Can you work these out from the model? Positions are in its coordinate system, mm. A direction names the side the tool comes from. Give positions to 0.01 mm unless a question says otherwise; leave off trailing zeros. Write each loop counter-clockwise with the first axis right and the second up, starting at its lowest first coordinate (ties: lowest second). Pieces come first, ordered by that corner, then holes. Notation, with made-up numbers: (-16, -9.5) -> (8, -9.5) arc R17 ccw to (8, 11.5) -> close; hole circle Ø5 at (-38.5, 8.25). An arc over 180 degrees is marked (long way). One line per item, written item: value.
Autodesk Inventor part; units mm, degrees
ref_plane "YZ Plane" through (0, 0, 0) normal (1, 0, 0) x (0, 1, 0)
ref_plane "XZ Plane" through (0, 0, 0) normal (0, 1, 0) x (-1, 0, 0)
ref_plane "XY Plane" through (0, 0, 0) normal (0, 0, 1) x (1, 0, 0)
sketch "Sketch1" plane through (0, 0, 0) normal (0, 0, 1) x (1, 0, 0)
  line L0 (-21.1, 10.5) -> (21.1, 10.5)
  line L1 (21.1, 10.5) -> (21.1, -10.5)
  line L2 (21.1, -10.5) -> (-21.1, -10.5)
  line L3 (-21.1, -10.5) -> (-21.1, 10.5)
  line L4 (-21.1, 10.5) -> (21.1, -10.5) construction
  line L5 (21.1, 10.5) -> (-21.1, -10.5) construction
  line L6 (31.1, 20.5) -> (-31.1, 20.5)
  line L7 (-31.1, 20.5) -> (-31.1, -20.5)
  line L8 (-31.1, -20.5) -> (31.1, -20.5)
  line L9 (31.1, -20.5) -> (31.1, 20.5)
  point P0 (0, 0)
  dimension "d0" = 42.2
  dimension "d1" = 21
  dimension "d2" = 10
extrude "Extrusion1" add sketch "Sketch1" along normal blind 9
sketch "Sketch2" plane through (-31.1, -20.5, 0) normal (0, -1, 0) x (1, 0, 0)
  line L0 (62.2, 9) -> (0, 9)
  line L1 (0, 9) -> (75, 9)
  line L2 (75, 9) -> (75, -11)
  line L3 (75, -11) -> (0, -11)
  line L4 (0, -11) -> (0, 9)
  point P0 (31.1, 0)
  dimension "d5" = 75
  dimension "d6" = 20
extrude "Extrusion2" add sketch "Sketch2" along normal blind 5
sketch "Sketch3" plane through (-31.1, 20.5, 0) normal (-1, 0, 0) x (0, 0, 1)
  line L0 (9, -46) -> (-11, -46)
  line L1 (9, -46) -> (-11, -46)
  line L2 (-11, -46) -> (-11, 14)
  line L3 (-11, 14) -> (9, 14)
  line L4 (9, 14) -> (9, -46)
  point P0 (0, -20.5)
  dimension "d9" = 20
  dimension "d10" = 60
extrude "Extrusion3" add sketch "Sketch3" along normal blind 5
sketch "Sketch4" plane through (-31.1, -25.5, 0) normal (0, -1, 0) x (1, 0, 0)
  line L0 (75, 9) -> (75, -11)
  line L1 (75, 2.3333) -> (-5, 2.3333)
  line L2 (-5, -11) -> (-5, 9)
  line L3 (75, -3.6667) -> (-5, -3.6667)
  line L4 (75, 9) -> (-5, 9)
  line L5 (75, 2.3333) -> (75, -3.6667)
  line L6 (-5, 2.3333) -> (-5, -3.6667)
  point P0 (31.1, 0)
  dimension "d13" = 6
  dimension "d14" = 6.6667
extrude "Extrusion4" add sketch "Sketch4" along normal blind 1.5 contours L0 L3 L2 L1
sketch "Sketch5" plane through (-36.1, 20.5, 0) normal (-1, 0, 0) x (0, 0, 1)
  line L0 (2.353, -47.5) -> (2.353, 14)
  line L1 (9, 14) -> (-11, 14)
  line L2 (2.3333, -47.5) -> (-3.6667, -47.5)
  line L3 (-3.6667, -47.5) -> (-3.6667, 14)
  line L4 (-3.6667, 14) -> (2.353, 14)
  line L5 (2.353, -47.5) -> (-3.6667, -47.5)
  point P0 (0, -20.5)
extrude "Extrusion5" add sketch "Sketch5" along normal blind 1.5
sketch "Sketch6" plane through (-37.6, 20.5, 0) normal (-1, 0, 0) x (0, 0, 1)
  line L0 (9, 14) -> (2.353, 14)
  line L1 (0, 0) -> (9, 0)
  line L2 (9, -46) -> (9, 14)
  line L3 (-11, 14) -> (-11, -46)
  point P0 (0, -20.5)
  point P1 (-1, 7)
  dimension "d19" = 14
  dimension "d20" = 20
  dimension "d21" = 10
  dimension "d22" = 7
hole "Hole1" at (-37.6, 27.5, -1) direction (1, 0, 0) diameter 6 end through all counterbore diameter 10 counterbore depth 1.5
sketch "Sketch7" plane through (-31.1, -27, 0) normal (0, -1, 0) x (1, 0, 0)
  line L0 (75, 2.3333) -> (75, 9)
  line L1 (62.2, 0) -> (62.2, 9)
  line L2 (75, -11) -> (-5, -11)
  line L3 (75, 9) -> (-5, 9)
  point P0 (31.1, 0)
  point P1 (68.6, -1)
  dimension "d30" = 12.8
  dimension "d31" = 20
  dimension "d32" = 10
  dimension "d33" = 6.4
hole "Hole2" at (37.5, -27, -1) direction (0, 1, 0) diameter 6 end through all counterbore diameter 10 counterbore depth 1.5
fillet "Fillet1" radius 2 9 edges at (31.1, 20.5, 4.5) (-33.6, 34.5, 9) (-33.6, 34.5, -11) (43.9, -23, 9) (43.9, -23, -11) (0, 10.5, 0) (0, -10.5, 0) (21.1, 0, 0) (-21.1, 0, 0)
properties part number "SuporteRJ45"
1) For faces 5 (the face through (43.33, -23.04, 8.4)), 6 (the face through (0, 14, 0)), 7 (the face through (31.1, -1, 4)), which set-ups out of +Z, -Z, +X, -X, +Y, -Y let a thin tool reach every point of the face, with its end or its side?
Answer list:
face 5: +Z, +X, +Y, -Y
face 6: -Z, +X, +Y
face 7: +Z, -Z, +X, +Y
2) If we section it at C-C (z = -1): Write out the boundary of the cut face in (x, y), and give its area (3 significant figures).
Answer list:
outline: (-37.6, -27) -> (32.5, -27) -> (32.5, -25.5) -> (34.5, -25.5) -> (34.5, -20.5) -> (-31.1, -20.5) -> (-31.1, 24.5) -> (-36.1, 24.5) -> (-36.1, 22.5) -> (-37.6, 22.5) -> close; (-37.6, 32.5) -> (-36.1, 32.5) -> (-36.1, 30.5) -> (-31.1, 30.5) -> (-31.1, 34.5) -> (-37.6, 34.5) -> close; (40.5, -25.5) -> (42.5, -25.5) -> (42.5, -27) -> (43.9, -27) -> (43.9, -20.5) -> (40.5, -20.5) -> close
area: 797 mm^2
3) We'd pull the mould along Y, two halves only. Please class faces 1 (the face through (21.1, 0, 5)), 2 (the face through (-14, -22, -11)), 3 (the face through (-21.67, 0.18, 0.6)), 4 (the face through (43, -27, -1)): released by +Y, released by -Y, zero draft, split by the parting line, or undercut.
Answer list:
face 1: undercut
face 2: zero draft
face 3: undercut
face 4: released by -Y
4) If we section it at B-B (x = 37.5): Write out the boundary of the cut face in (y, z).
Answer list:
outline: (-25.5, -11) -> (-20.5, -11) -> (-20.5, -4) -> (-25.5, -4) -> close; (-25.5, 2) -> (-20.5, 2) -> (-20.5, 9) -> (-25.5, 9) -> close
5) If we section it at A-A (y = 27.5): Write out the boundary of the cut face in (x, z).
Answer list:
outline: (-36.1, -11) -> (-31.1, -11) -> (-31.1, -4) -> (-36.1, -4) -> close; (-36.1, 2) -> (-31.1, 2) -> (-31.1, 9) -> (-36.1, 9) -> close
6) I need wall thicknesses on L1, parallel to Y at x = -6, z = 3.25; L2, parallel to X at y = -23.95, z = -1; L3, parallel to X at y = -9.5, z = 5.75. Which ranges of each line are inside material? Lowest first, please.
Answer list:
L1: y = -25.5 to -10.5, 10.5 to 20.5
L2: x = -37.6 to 34.5, 40.5 to 43.9
L3: x = -36.1 to -21.1, 21.1 to 31.1
7) Will these pins go through, and if not, where does the flat tip stop? pin 1 (3.5 mm diameter, centred on y = 27.5, z = -1, fed in from +X); pin 2 (8 mm diameter, centred on x = 23.5, z = -1.5, fed in from +Y); pin 3 (5.5 mm diameter, centred on x = -4.5, z = 6.5, fed in from -Y); pin 4 (3 mm diameter, centred on y = 16, z = -9, fed in from +X).
Answer list:
pin 1: passes through
pin 2: stops at y = 20.5
pin 3: stops at y = -25.5
pin 4: stops at x = -31.1
8) If we section it at D-D (y = -16.5): Write out the boundary of the cut face in (x, z).
Answer list:
outline: (-37.6, -3.67) -> (-36.1, -3.67) -> (-36.1, -11) -> (-31.1, -11) -> (-31.1, 0) -> (31.1, 0) -> (31.1, 9) -> (-36.1, 9) -> (-36.1, 2.35) -> (-37.6, 2.35) -> close
